Verification items for the finished model (mm, model axes). Face numbers are marked on the shaded views. A direction names the side the tool comes from. Coordinates: 2 decimals unless noted, no trailing zeros. Order: outer loops, then holes, each group sorted by start corner. A loop starts at its lowest first (then second) coordinate and runs counter-clockwise, first axis right, second up.
Q1. Depth check by flat-ended pin: P1, Ø8, axis at x = 8.5, z = 8.5, coming from the +Y side; P2, Ø1.5, axis at x = 18.5, z = 5.5, coming from the +Y side; P3, Ø5.5, axis at y = 10.5, z = 15, coming from the +X side. Enter the tip coordinate at first touch or a pass-through.
Q2. Cross-section at C-C, the plane y = 20.5. Record the boundary of the cut face in (x, z), and give its area (3 significant figures).
Q3. Cross-section at D-D, the plane x = 0.5. Record the boundary of the cut face in (y, z).
Q4. Set-up check for the marked faces 1, 2 and 3: record each of +Z, -Z, +X, -X, +Y, -Y from which the full face is reachable in a straight line by a thin tool's end or side.
Q5. Cross-section at B-B, the plane z = -15. Record the boundary of the cut face in (x, y), and give its area (3 significant figures).
Q6. Cross-section at A-A, the plane y = 11.5. Record the boundary of the cut face in (x, z), and give its area (3 significant figures).
Q7. Thickness scan on line 1 (Z direction, x = -5, y = 4.5); line 2 (Y direction, x = 8, z = 15); line 3 (Y direction, x = 21, z = -12). Record the ranges inside material, lowest first.
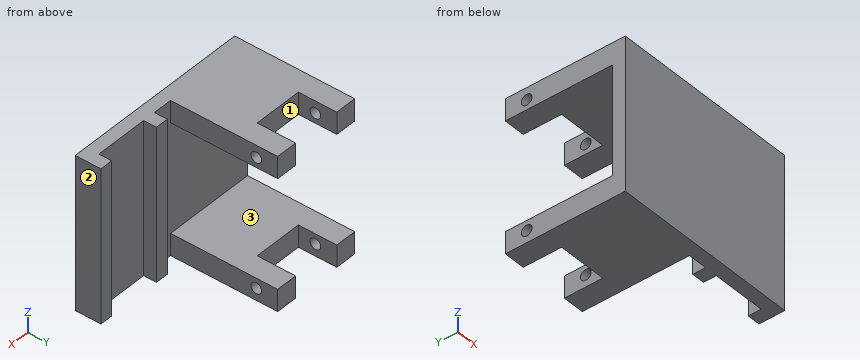
from build123d import *

# Parameters (mm, degrees)
SKETCH1_W           = 36.5
SKETCH1_H           = 35.6
BOSS_EXTRUDE1_DEPTH = 3
SKETCH2_W           = 3
SKETCH2_H           = 5.1
BOSS_EXTRUDE2_DEPTH = 23
SKETCH3_R           = 1.35
CUT_EXTRUDE1_DEPTH  = 37.5
SKETCH4_W           = 35.6
SKETCH4_H           = 3
BOSS_EXTRUDE3_DEPTH = 12.5
SKETCH5_W           = 3
SKETCH5_H           = 35.6
BOSS_EXTRUDE4_DEPTH = 6
SKETCH9_W           = 21.5
SKETCH9_H           = 5.1
BOSS_EXTRUDE6_DEPTH = 25
SKETCH10_R          = 1.25
CUT_EXTRUDE4_DEPTH  = 45.5
SKETCH11_W          = 3
SKETCH11_H          = 23
CUT_EXTRUDE5_DEPTH  = 36.6
SKETCH12_W          = 11.5
SKETCH12_H          = 8.963057692
CUT_EXTRUDE6_DEPTH  = 36.6
SKETCH13_W          = 3
SKETCH13_H          = 35.6
BOSS_EXTRUDE7_DEPTH = 3
SKETCH15_W          = 23
SKETCH15_H          = 35.6
CUT_EXTRUDE9_DEPTH  = 6


with BuildPart() as part:
    # Sketch1 → Boss-Extrude1 (new body)
    with BuildSketch(Plane(origin=(0, 0, 0), x_dir=(1, 0, 0), z_dir=(0, 1, 0))):
        Rectangle(SKETCH1_W, SKETCH1_H)
    extrude(amount=BOSS_EXTRUDE1_DEPTH)

    # Sketch2 → Boss-Extrude2 (add)
    with BuildSketch(Plane(origin=(0, 3, 0), x_dir=(1, 0, 0), z_dir=(0, 1, 0))):
        with Locations((-16.75, 15.25)):
            Rectangle(SKETCH2_W, SKETCH2_H)
        with Locations((-16.75, -15.25)):
            Rectangle(SKETCH2_W, SKETCH2_H)
        with Locations((16.75, 15.25)):
            Rectangle(SKETCH2_W, SKETCH2_H)
        with Locations((16.75, -15.25)):
            Rectangle(SKETCH2_W, SKETCH2_H)
    extrude(amount=BOSS_EXTRUDE2_DEPTH)

    # Sketch3 → Cut-Extrude1 (cut, through all)
    with BuildSketch(Plane(origin=(18.25, 0, 0), x_dir=(0, 0, -1), z_dir=(1, 0, 0))):
        with Locations((-15, 23)):
            Circle(SKETCH3_R)
        with Locations((15, 23)):
            Circle(SKETCH3_R)
    extrude(amount=-CUT_EXTRUDE1_DEPTH, mode=Mode.SUBTRACT)

    # Sketch4 → Boss-Extrude3 (add)
    with BuildSketch(Plane(origin=(18.25, 0, 0), x_dir=(0, 0, -1), z_dir=(1, 0, 0))):
        with Locations((0, 1.5)):
            Rectangle(SKETCH4_W, SKETCH4_H)
    boss_extrude3 = extrude(amount=BOSS_EXTRUDE3_DEPTH)

    # Mirror1: Boss-Extrude3 across plane
    add(boss_extrude3.mirror(Plane(origin=(0, 0, 0), x_dir=(0, 0, 1), z_dir=(1, 0, 0))))

    # Sketch5 → Boss-Extrude4 (add)
    with BuildSketch(Plane.XZ):
        with Locations((32.25, 0)):
            Rectangle(SKETCH5_W, SKETCH5_H)
    boss_extrude4 = extrude(amount=-BOSS_EXTRUDE4_DEPTH)

    # Mirror2: Boss-Extrude4 across plane
    add(boss_extrude4.mirror(Plane(origin=(0, 0, 0), x_dir=(0, 0, 1), z_dir=(1, 0, 0))))

    # Sketch9 → Boss-Extrude6 (add)
    with BuildSketch(Plane(origin=(0, 3, 0), x_dir=(1, 0, 0), z_dir=(0, 1, 0))):
        with Locations((0, 15.25)):
            Rectangle(SKETCH9_W, SKETCH9_H)
        with Locations((0, -15.25)):
            Rectangle(SKETCH9_W, SKETCH9_H)
    extrude(amount=BOSS_EXTRUDE6_DEPTH)

    # Sketch10 → Cut-Extrude4 (cut, through all)
    with BuildSketch(Plane(origin=(10.75, 0, 0), x_dir=(0, 0, -1), z_dir=(1, 0, 0))):
        with Locations((15, 23)):
            Circle(SKETCH10_R)
        with Locations((-15, 23)):
            Circle(SKETCH10_R)
    extrude(amount=-CUT_EXTRUDE4_DEPTH, mode=Mode.SUBTRACT)

    # Sketch11 → Cut-Extrude5 (cut, through all)
    with BuildSketch(Plane(origin=(0, 0, -17.8), x_dir=(-1, 0, 0), z_dir=(0, 0, -1))):
        with Locations((-16.75, 14.5)):
            Rectangle(SKETCH11_W, SKETCH11_H)
        with Locations((16.75, 14.5)):
            Rectangle(SKETCH11_W, SKETCH11_H)
    extrude(amount=-CUT_EXTRUDE5_DEPTH, mode=Mode.SUBTRACT)

    # Sketch12 → Cut-Extrude6 (cut, through all)
    with BuildSketch(Plane(origin=(0, 0, -17.8), x_dir=(-1, 0, 0), z_dir=(0, 0, -1))):
        with Locations((0, 23.518471154)):
            Rectangle(SKETCH12_W, SKETCH12_H)
    extrude(amount=-CUT_EXTRUDE6_DEPTH, mode=Mode.SUBTRACT)

    # Sketch13 → Boss-Extrude7 (add)
    with BuildSketch(Plane(origin=(0, 3, 0), x_dir=(1, 0, 0), z_dir=(0, 1, 0))):
        with Locations((16.75, 0)):
            Rectangle(SKETCH13_W, SKETCH13_H)
    extrude(amount=BOSS_EXTRUDE7_DEPTH)

    # Sketch15 → Cut-Extrude9 (cut)
    with BuildSketch(Plane(origin=(0, 6, 0), x_dir=(1, 0, 0), z_dir=(0, 1, 0))):
        with Locations((-22.25, 0)):
            Rectangle(SKETCH15_W, SKETCH15_H)
    extrude(amount=-CUT_EXTRUDE9_DEPTH, mode=Mode.SUBTRACT)


solid = part.part
Check values:
1. P1: stops at y = 3
1. P2: stops at y = 6
1. P3: stops at x = 10.75
2. outline: (-10.75, -17.8) - (-5.75, -17.8) - (-5.75, -12.7) - (-10.75, -12.7) - close; (-10.75, 12.7) - (-5.75, 12.7) - (-5.75, 17.8) - (-10.75, 17.8) - close; (5.75, -17.8) - (10.75, -17.8) - (10.75, -12.7) - (5.75, -12.7) - close; (5.75, 12.7) - (10.75, 12.7) - (10.75, 17.8) - (5.75, 17.8) - close
2. area: 102 mm2
3. outline: (0, -17.8) - (19.04, -17.8) - (19.04, -12.7) - (3, -12.7) - (3, 12.7) - (19.04, 12.7) - (19.04, 17.8) - (0, 17.8) - close
4. face 1: +Z, -Z, +Y
4. face 2: +Z, -Z, +X, +Y, -Y
4. face 3: -X, +Y
5. outline: (-10.75, 0) - (33.75, 0) - (33.75, 6) - (30.75, 6) - (30.75, 3) - (18.25, 3) - (18.25, 6) - (15.25, 6) - (15.25, 3) - (10.75, 3) - (10.75, 21.75) - (5.75, 21.75) - (5.75, 19.04) - (-5.75, 19.04) - (-5.75, 21.75) - (-10.75, 21.75) - close; (-10.75, 24.25) - (-5.75, 24.25) - (-5.75, 28) - (-10.75, 28) - close; (5.75, 24.25) - (10.75, 24.25) - (10.75, 28) - (5.75, 28) - close
5. area: 561 mm2
6. outline: (-10.75, -17.8) - (10.75, -17.8) - (10.75, -12.7) - (-10.75, -12.7) - close; (-10.75, 12.7) - (10.75, 12.7) - (10.75, 17.8) - (-10.75, 17.8) - close
6. area: 219 mm2
7. line 1: z = -17.8 to -12.7, 12.7 to 17.8
7. line 2: y = 0 to 21.75, 24.25 to 28
7. line 3: y = 0 to 3
